Here's how the part is built. I have some questions about the finished solid (model axes, mm). Give positions to 0.01 mm unless a question says otherwise; leave off trailing zeros. Loops run counter-clockwise (first coordinate to the right, second up) from the corner with the lowest first, then second, coordinate; pieces in that order, holes last. Notation, with made-up numbers: M -38.75,20.25 L -34.75,20.25 A8 ccw -34.75,24.25 Z; hole C -35.75,13 d8. An arc over 180 degrees is marked long. Write item = value, one per line. Start each with the question number.
```python
from build123d import *

# Parameters (mm, degrees)
F0_W     = 88.9
F0_H     = 25.4
F1_DEPTH = 12.7
F3_DEPTH = 25.4
F4_R     = 2.54
F5_R     = 2.1209
F6_DEPTH = 26.162


with BuildPart() as f1:
    # F0 (on Front) → F1 (new body)
    with BuildSketch(Plane.XZ):
        with Locations((44.45, 12.7)):
            Rectangle(F0_W, F0_H)
    extrude(amount=F1_DEPTH)

    # F2 (on face) → F3 (cut)
    with BuildSketch(Plane(origin=(0, 0, 0), x_dir=(1, 0, 0), z_dir=(0, 0, -1))):
        Polygon((0, 6.35), (44.45, 12.7), (0, 12.7), align=None)
    extrude(amount=-F3_DEPTH, mode=Mode.SUBTRACT)

    # F4
    f4_edges = [f1.edges().sort_by_distance(p)[0] for p in [
        (0, 0, 12.7),
        (0, -6.35, 12.7),
        (88.9, 0, 12.7),
        (66.675, -12.7, 0),
        (66.675, -12.7, 25.4),
        (88.9, -12.7, 12.7),
        (44.45, -12.7, 12.7),
    ]]
    fillet(f4_edges, radius=F4_R)

    # F5 (on face) → F6 (cut)
    with BuildSketch(Plane.XY.offset(25.4)):
        with Locations((82.55, -2.54)):
            Circle(F5_R)
        with Locations((6.6528792481, -2.54)):
            Circle(F5_R)
    extrude(amount=-F6_DEPTH, mode=Mode.SUBTRACT)


solid = f1.part
```
Q1. If we section it at C-C, the plane y = -1.5: List the corners of the cut face in (x, z) for me, then the cut area to 3 significant figures.
Q2. Will these pins go through, and if not, where does the flat tip stop? pin 1 (5 mm diameter, centred on x = 82.55, y = -2.54, fed in from +Z); pin 2 (1 mm diameter, centred on x = 19.5, z = 5.5, fed in from -Y); pin 3 (5 mm diameter, centred on x = 9, z = 10.5, fed in from -Y); pin 4 (10 mm diameter, centred on x = 31.5, z = 22.5, fed in from -Y).
Q3. If we section it at A-A, the plane x = 82.55: List the corners of the cut face in (y, z) for me, then the cut area to 3 significant figures.
Q4. If I drill on line 1 along Y through (x, z) = (82.55, 5.5); line 2 along X through (y, z) = (-1.5, 19.5); line 3 along X through (y, z) = (-1, 13), over which ranges is the centre line in solid material (lowest first)?
Q5. If we section it at D-D, the plane x = 33: List the corners of the cut face in (y, z) for me.
Q6. If we section it at B-B, the plane z = 14.25: List the corners of the cut face in (x, y) for me.
Q7. We'd pull the mould along X, two halves only. Please class faces 1 (the cylindrical face through (80.43, -2.45, 12.88)), 2 (the flat face through (44, -5, 25.4)), 3 (the cylindrical face through (0.724, -0.764, 12.878)), 4 (the cylindrical face through (88.136, -0.724, 12.878)): pulls with the +X half, pulls with the -X half, needs draft (parallel to the pull), parting line crosses it, or undercut.
Resolved:
q1.outline = M 0.22,0 L 4.8,0 L 4.8,25.4 L 0.22,25.4 Z; M 8.5,0 L 80.7,0 L 80.7,25.4 L 8.5,25.4 Z; M 84.4,0 L 88.68,0 L 88.68,25.4 L 84.4,25.4 Z
q1.area = 2,060 mm²
q2.pin_1 = 25.4
q2.pin_2 = -9.21
q2.pin_3 = -7.99
q2.pin_4 = -11.56
q3.outline = M -12.7,2.54 A2.54 ccw -10.16,0 L -4.66,0 L -4.66,25.4 L -10.16,25.4 A2.54 ccw -12.7,22.86 Z; M -0.42,0 L 0,0 L 0,25.4 L -0.42,25.4 Z
q3.area = 212 mm²
q4.line_1 = -12.7 to -4.66, -0.42 to 0
q4.line_2 = 0.22 to 4.8, 8.5 to 80.7, 84.4 to 88.68
q4.line_3 = 0.52 to 5.19, 8.11 to 81.09, 84.01 to 88.38
q5.outline = M -11.06,0.17 A2.54 ccw -10.16,0 L 0,0 L 0,25.4 L -10.16,25.4 A2.54 ccw -11.06,25.23 Z
q6.outline = M 0,-4.15 A2.54 ccw 2.18,-6.66 L 44.27,-12.67 A2.54 ccw 44.63,-12.7 L 86.36,-12.7 A2.54 ccw 88.9,-10.16 L 88.9,-2.54 A2.54 ccw 86.36,0 L 2.54,0 A2.54 ccw 0,-2.54 Z; hole C 6.65,-2.54 d4.24; hole C 82.55,-2.54 d4.24
q7.face_1 = undercut
q7.face_2 = needs draft
q7.face_3 = pulls with the -X half
q7.face_4 = pulls with the +X half
